Autodesk Inventor part; units mm, degrees
ref_plane "YZ Plane" through (0, 0, 0) normal (1, 0, 0) x (0, 1, 0)
ref_plane "XZ Plane" through (0, 0, 0) normal (0, 1, 0) x (-1, 0, 0)
ref_plane "XY Plane" through (0, 0, 0) normal (0, 0, 1) x (1, 0, 0)
sketch "スケッチ1" plane through (0, 0, 0) normal (1, 0, 0) x (0, 1, 0)
  line L0 (0, 0) -> (20, 0)
  line L1 (20, 0) -> (20, -20)
  line L2 (20, -20) -> (0, -20)
  line L3 (0, -20) -> (0, 0)
  line L4 (102.9471, -35) -> (9.6, -35)
  line L5 (9.6, -35) -> (9.6, -45.8)
  line L6 (9.6, -45.8) -> (102.9471, -45.8)
  line L7 (102.9471, -45.8) -> (102.9471, -35)
  circle A0 centre (14, -10) radius 1.5
  circle A1 centre (6, -10) radius 1.5
  line L8 (20, -45.8) -> (0, -45.8)
  line L9 (0, -45.8) -> (0, -50.8)
  line L10 (0, -50.8) -> (20, -50.8)
  line L11 (20, -50.8) -> (20, -45.8)
  line L12 (0, -20) -> (0, -45.8)
  line L13 (20, -20) -> (20, -35)
  dimension "d0" = 20
  dimension "d1" = 20
  dimension "d2" = 10.8
  dimension "d3" = 9.6
  dimension "d4" = 15
  dimension "d5" = 3
  dimension "d6" = 3
  dimension "d7" = 10
  dimension "d8" = 10
  dimension "d9" = 6
  dimension "d10" = 8
  dimension "d11" = 5
  dimension "d12" = 20
  dimension "d13" = 0
extrude "押し出し1" add sketch "スケッチ1" along normal blind 6 contours L0 L1 L2 L3 | L2 L13 L4 L5 L8 L12 | L8 L6 L11 L10 L9
fillet "フィレット1" radius 2 6 edges at (3, 0, 0) (3, 20, 0) (3, 20, -35) (3, 20, -45.8) (3, 20, -50.8) (3, 0, -50.8)
sketch "スケッチ2" plane through (6, 0, 0) normal (1, 0, 0) x (0, 0, -1)
  arc A0 (48.8, 0) -> (50.8, 2) centre (48.8, 2) ccw
  line L0 (50.8, 2) -> (50.8, 18)
  arc A1 (50.8, 18) -> (48.8, 20) centre (48.8, 18) ccw
  line L1 (48.8, 20) -> (47.8, 20)
  arc A2 (47.8, 20) -> (45.8, 18) centre (47.8, 18) ccw
  line L2 (45.8, 18) -> (45.8, 9.6)
  line L3 (45.8, 9.6) -> (35, 9.6)
  line L4 (35, 9.6) -> (35, 18)
  arc A3 (35, 18) -> (33, 20) centre (33, 18) ccw
  line L5 (33, 20) -> (2, 20)
  arc A4 (2, 20) -> (0, 18) centre (2, 18) ccw
  line L6 (0, 18) -> (0, 2)
  arc A5 (0, 2) -> (2, 0) centre (2, 2) ccw
  line L7 (2, 0) -> (48.8, 0)
  circle A6 centre (10, 6) radius 1.5
  circle A7 centre (10, 14) radius 1.5
  point P0 (0, 0)
equation "\"d12\" = d1"
properties part number "base_weel-v2-POM-pc-F-1" material "ABS プラスチック"
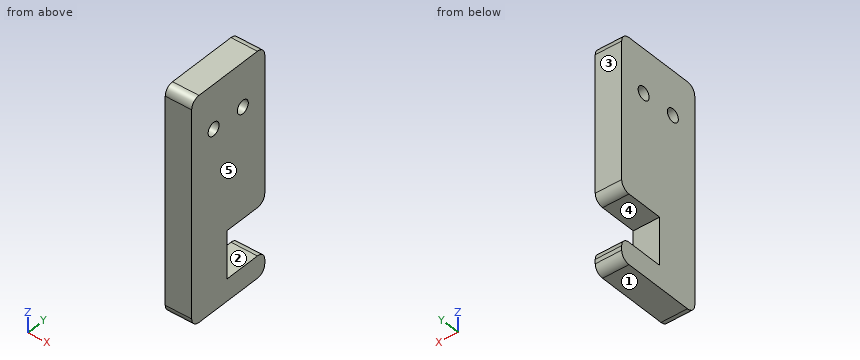
CAD build for the part. Positions are in the model's coordinates, mm. Face numbers are marked on the shaded views. A direction names the side the tool comes from. Coordinates: 2 decimals unless noted, no trailing zeros. Write each loop counter-clockwise with the first axis right and the second up, starting at its lowest first coordinate (ties: lowest second). Pieces come first, ordered by that corner, then holes. Notation, with made-up numbers: (9, 40.25) -> (60, 40.25) arc R14 ccw to (60, 53.25) -> close; hole circle Ø11 at (-28.75, -24.5). An arc over 180 degrees is marked (long way). Use CSV: the item, a comma, the result in double quotes. Start each with the question number.
Item 1: Wall check: probe 1 along Z at (x, y) = (2.95, 10.75); probe 2 along Z at (x, y) = (4.7, 14); probe 3 along Z at (x, y) = (0.4, 15.25). Give the ranges that are in metal, low to high.
Item 2: Two-plate mould, pull along Z, no slides. Class the marked faces 1, 2 and 3: +Z half, -Z half, draft (parallel to the pull), parting line (faces both ways), or undercut.
Item 3: Band-saw the part on C-C, the plane y = 14. Write the cut outline in (x, z).
Item 4: Band-saw the part on D-D, the plane z = -10.5. Write the cut outline in (x, y), plus the area to 3 significant figures.
Item 5: Drop a flat-ended pin along its axis: P1, Ø2, axis at y = 4.5, z = -33.5, coming from the -X side. Give the stop position or say it passes through.
Item 6: Band-saw the part on B-B, the plane x = 2.6. Write the cut outline in (y, z), plus the area to 3 significant figures.
Item 7: Band-saw the part on A-A, the plane y = 6. Write the cut outline in (x, z).
Item 8: Tool access for the marked faces 4 and 5: list every direction of +Z, -Z, +X, -X, +Y, -Y with a clear straight run to the whole face (end or side of a thin tool).
Response values:
1,probe 1,"z = -50.8 to -45.8, -35 to 0"
1,probe 2,"z = -50.8 to -45.8, -35 to -11.5, -8.5 to 0"
1,probe 3,"z = -50.8 to -45.8, -35 to -10.83, -9.17 to 0"
2,face 1,"-Z half"
2,face 2,"undercut"
2,face 3,"draft"
3,outline,"(0, -50.8) -> (6, -50.8) -> (6, -45.8) -> (0, -45.8) -> close; (0, -35) -> (6, -35) -> (6, -11.5) -> (0, -11.5) -> close; (0, -8.5) -> (6, -8.5) -> (6, 0) -> (0, 0) -> close"
4,outline,"(0, 0) -> (6, 0) -> (6, 4.59) -> (0, 4.59) -> close; (0, 7.41) -> (6, 7.41) -> (6, 12.59) -> (0, 12.59) -> close; (0, 15.41) -> (6, 15.41) -> (6, 20) -> (0, 20) -> close"
4,area,"86.1 mm2"
5,P1,"stops at x = 0"
6,outline,"(0, -48.8) arc R2 ccw to (2, -50.8) -> (18, -50.8) arc R2 ccw to (20, -48.8) -> (20, -47.8) arc R2 ccw to (18, -45.8) -> (9.6, -45.8) -> (9.6, -35) -> (18, -35) arc R2 ccw to (20, -33) -> (20, -2) arc R2 ccw to (18, 0) -> (2, 0) arc R2 ccw to (0, -2) -> close; hole circle Ø3 at (6, -10); hole circle Ø3 at (14, -10)"
6,area,"884 mm2"
7,outline,"(0, -50.8) -> (6, -50.8) -> (6, -11.5) -> (0, -11.5) -> close; (0, -8.5) -> (6, -8.5) -> (6, 0) -> (0, 0) -> close"
8,face 4,"+X, -X, +Y"
8,face 5,"+Z, -Z, +X, +Y, -Y"
